Here's how the part is built. I have some questions about the finished solid (model axes, mm). Face numbers are marked on the shaded views. Coordinates: 2 decimals unless noted, no trailing zeros. Answer in a Markdown table with one row per item. Add a question column.
Item 1: Thinking about a two-plate mould opening in Z: for the marked faces 1 and 2, which applies, +Z half, -Z half, draft (parallel to the pull), parting line (faces both ways), or undercut?
Item 2: Will these pins go through, and if not, where does the flat tip stop? pin 1 Ø1.8 at (x, y) = (-30.08, -16.5) entering from -Z; pin 2 Ø3 at (x, y) = (28.5, 15) entering from -Z; pin 3 Ø3 at (x, y) = (-30.08, 16.5) entering from -Z.
Item 3: If I drill on line 1 along Y through (x, z) = (0, 0.2); line 2 along X through (y, z) = (-14, -0.3); line 3 along Y through (x, z) = (29.5, -0.4), over which ranges is the centre line in solid material (lowest first)? Write a range as from..to.
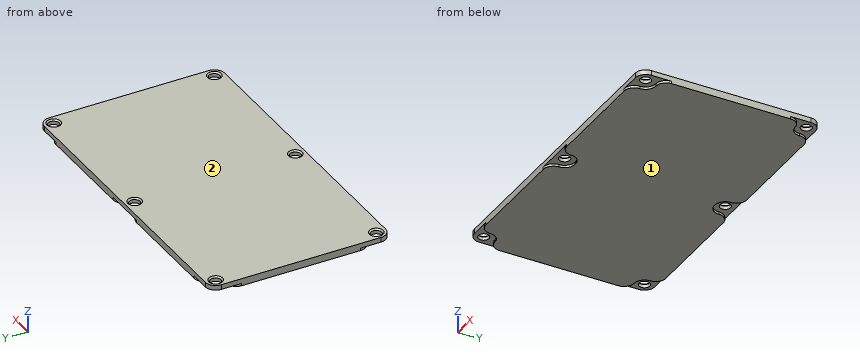
```python
from build123d import *

# Parameters (mm, degrees)
SKETCH_1_W          = 64
SKETCH_1_H          = 37
EXTRUDE_1_DEPTH     = 1
SKETCH_2_W          = 4.2
SKETCH_2_H          = 28.6
SKETCH_2_W_2        = 25.55
SKETCH_2_H_2        = 4.2
SKETCH_2_W_3        = 4.5
EXTRUDE_2_DEPTH     = 0.5
FILLET_1_R          = 2.1
CUT_EXTRUDE_1_REACH = 38.993
SKETCH_3_R          = 1.1
CHAMFER_1_SIZE      = 0.3


with BuildPart() as part:
    # 스케치1 → 보스-돌출1 (new body)
    with BuildSketch(Plane.XY):
        Rectangle(SKETCH_1_W, SKETCH_1_H)
    extrude(amount=EXTRUDE_1_DEPTH)

    # 스케치2 → 보스-돌출2 (add)
    with BuildSketch(Plane(origin=(0, 0, 0), x_dir=(-1, 0, 0), z_dir=(0, 0, -1))):
        with Locations((-29.9, 0)):
            Rectangle(SKETCH_2_W, SKETCH_2_H)
        with Locations((-15.025, 0)):
            Rectangle(SKETCH_2_W_2, SKETCH_2_H)
        with Locations((-15.025, 16.4)):
            Rectangle(SKETCH_2_W_2, SKETCH_2_H_2)
        with Locations((-15.025, -16.4)):
            Rectangle(SKETCH_2_W_2, SKETCH_2_H_2)
        with Locations((15.025, 0)):
            Rectangle(SKETCH_2_W_2, SKETCH_2_H)
        with Locations((15.025, 16.4)):
            Rectangle(SKETCH_2_W_2, SKETCH_2_H_2)
        Rectangle(SKETCH_2_W_3, SKETCH_2_H)
        with Locations((29.9, 0)):
            Rectangle(SKETCH_2_W, SKETCH_2_H)
        with Locations((15.025, -16.4)):
            Rectangle(SKETCH_2_W_2, SKETCH_2_H_2)
    extrude(amount=EXTRUDE_2_DEPTH)

    # 필렛1
    # the kernel refuses this fillet: 2.1 mm, written as the material it adds along each edge
    with BuildSketch(Plane(origin=(27.8, -14.3, 5.25), x_dir=(0, -1, 0), z_dir=(0, 0, -1))) as fillet_1_piece_1_section:
        with BuildLine():
            CenterArc((FILLET_1_R, -FILLET_1_R), FILLET_1_R, 90, 90)
            Line((0, -FILLET_1_R), (0, 0))
            Line((0, 0), (FILLET_1_R, 0))
        make_face()
    fillet_1_piece_1 = extrude(amount=5.75, mode=Mode.PRIVATE)
    fillet_1_piece_1 = split(fillet_1_piece_1, bisect_by=Plane(origin=(28.269072672, -14.769072672, 1), z_dir=(0, 0, -1)), keep=Keep.TOP, mode=Mode.PRIVATE)
    add(fillet_1_piece_1)
    with BuildSketch(Plane(origin=(-2.25, -14.3, 5.25), x_dir=(0, -1, 0), z_dir=(0, 0, -1))) as fillet_1_piece_2_section:
        with BuildLine():
            CenterArc((FILLET_1_R, -FILLET_1_R), FILLET_1_R, 90, 90)
            Line((0, -FILLET_1_R), (0, 0))
            Line((0, 0), (FILLET_1_R, 0))
        make_face()
    fillet_1_piece_2 = extrude(amount=5.75, mode=Mode.PRIVATE)
    fillet_1_piece_2 = split(fillet_1_piece_2, bisect_by=Plane(origin=(-1.780927328, -14.769072672, 1), z_dir=(0, 0, -1)), keep=Keep.TOP, mode=Mode.PRIVATE)
    add(fillet_1_piece_2)
    with BuildSketch(Plane(origin=(2.25, -14.3, 5.25), x_dir=(-1, 0, 0), z_dir=(0, 0, -1))) as fillet_1_piece_3_section:
        with BuildLine():
            CenterArc((FILLET_1_R, -FILLET_1_R), FILLET_1_R, 90, 90)
            Line((0, -FILLET_1_R), (0, 0))
            Line((0, 0), (FILLET_1_R, 0))
        make_face()
    fillet_1_piece_3 = extrude(amount=5.75, mode=Mode.PRIVATE)
    fillet_1_piece_3 = split(fillet_1_piece_3, bisect_by=Plane(origin=(1.780927328, -14.769072672, 1), z_dir=(0, 0, -1)), keep=Keep.TOP, mode=Mode.PRIVATE)
    add(fillet_1_piece_3)
    with BuildSketch(Plane(origin=(-27.8, -14.3, 5.25), x_dir=(-1, 0, 0), z_dir=(0, 0, -1))) as fillet_1_piece_4_section:
        with BuildLine():
            CenterArc((FILLET_1_R, -FILLET_1_R), FILLET_1_R, 90, 90)
            Line((0, -FILLET_1_R), (0, 0))
            Line((0, 0), (FILLET_1_R, 0))
        make_face()
    fillet_1_piece_4 = extrude(amount=5.75, mode=Mode.PRIVATE)
    fillet_1_piece_4 = split(fillet_1_piece_4, bisect_by=Plane(origin=(-28.269072672, -14.769072672, 1), z_dir=(0, 0, -1)), keep=Keep.TOP, mode=Mode.PRIVATE)
    add(fillet_1_piece_4)
    with BuildSketch(Plane(origin=(27.8, 14.3, 0), x_dir=(1, 0, 0), z_dir=(0, 0, -1)), Plane(origin=(-27.8, 14.3, 0), x_dir=(0, 1, 0), z_dir=(0, 0, -1))) as fillet_1_piece_5:
        with BuildLine():
            CenterArc((FILLET_1_R, -FILLET_1_R), FILLET_1_R, 90, 90)
            Line((0, -FILLET_1_R), (0, 0))
            Line((0, 0), (FILLET_1_R, 0))
        make_face()
    extrude(amount=0.5)
    with BuildSketch(Plane(origin=(-2.25, 14.3, 0), x_dir=(0, 1, 0), z_dir=(0, 0, -1)), Plane(origin=(2.25, 14.3, 0), x_dir=(-1, 0, 0), z_dir=(0, 0, -1))) as fillet_1_piece_6:
        with BuildLine():
            CenterArc((FILLET_1_R, FILLET_1_R), FILLET_1_R, 180, 90)
            Line((0, FILLET_1_R), (0, 0))
            Line((0, 0), (FILLET_1_R, 0))
        make_face()
    extrude(amount=0.5)
    # the kernel refuses this fillet: 2.1 mm, written as the material it takes off along each edge
    with BuildSketch(Plane(origin=(32, -18.5, -5.25), x_dir=(-1, 0, 0), z_dir=(0, 0, 1)), Plane(origin=(32, 18.5, -5.25), x_dir=(0, -1, 0), z_dir=(0, 0, 1))) as fillet_1_2_piece_1:
        with BuildLine():
            CenterArc((FILLET_1_R, -FILLET_1_R), FILLET_1_R, 90, 90)
            Line((0, -FILLET_1_R), (0, 0))
            Line((0, 0), (FILLET_1_R, 0))
        make_face()
    extrude(amount=11.5, mode=Mode.SUBTRACT)
    with BuildSketch(Plane(origin=(32, -14.3, 0), x_dir=(0, 1, 0), z_dir=(0, 0, -1)), Plane(origin=(27.8, 18.5, 0), x_dir=(-1, 0, 0), z_dir=(0, 0, -1)), Plane(origin=(-2.25, 18.5, 0), x_dir=(-1, 0, 0), z_dir=(0, 0, -1)), Plane(origin=(2.25, -18.5, 0), x_dir=(1, 0, 0), z_dir=(0, 0, -1)), Plane(origin=(-27.8, -18.5, 0), x_dir=(1, 0, 0), z_dir=(0, 0, -1)), Plane(origin=(-32, 14.3, 0), x_dir=(0, -1, 0), z_dir=(0, 0, -1))) as fillet_1_2_piece_2:
        with BuildLine():
            CenterArc((FILLET_1_R, -FILLET_1_R), FILLET_1_R, 90, 90)
            Line((0, -FILLET_1_R), (0, 0))
            Line((0, 0), (FILLET_1_R, 0))
        make_face()
    extrude(amount=5.75, mode=Mode.SUBTRACT)
    with BuildSketch(Plane(origin=(-32, -14.3, 0), x_dir=(0, 1, 0), z_dir=(0, 0, -1)), Plane(origin=(27.8, -18.5, 0), x_dir=(-1, 0, 0), z_dir=(0, 0, -1)), Plane(origin=(-2.25, -18.5, 0), x_dir=(-1, 0, 0), z_dir=(0, 0, -1)), Plane(origin=(2.25, 18.5, 0), x_dir=(1, 0, 0), z_dir=(0, 0, -1)), Plane(origin=(-27.8, 18.5, 0), x_dir=(1, 0, 0), z_dir=(0, 0, -1)), Plane(origin=(32, 14.3, 0), x_dir=(0, -1, 0), z_dir=(0, 0, -1))) as fillet_1_2_piece_3:
        with BuildLine():
            CenterArc((FILLET_1_R, FILLET_1_R), FILLET_1_R, 180, 90)
            Line((0, FILLET_1_R), (0, 0))
            Line((0, 0), (FILLET_1_R, 0))
        make_face()
    extrude(amount=5.75, mode=Mode.SUBTRACT)
    with BuildSketch(Plane(origin=(-32, -18.5, -5.25), x_dir=(1, 0, 0), z_dir=(0, 0, 1)), Plane(origin=(-32, 18.5, -5.25), x_dir=(0, -1, 0), z_dir=(0, 0, 1))) as fillet_1_2_piece_4:
        with BuildLine():
            CenterArc((FILLET_1_R, FILLET_1_R), FILLET_1_R, 180, 90)
            Line((0, FILLET_1_R), (0, 0))
            Line((0, 0), (FILLET_1_R, 0))
        make_face()
    extrude(amount=11.5, mode=Mode.SUBTRACT)

    # 스케치3 → 컷-돌출1 (cut, up to next)
    with BuildSketch(Plane.XY.offset(1), mode=Mode.PRIVATE) as cut_extrude_1_sk1:
        with Locations((-30.08, 16.5)):
            Circle(SKETCH_3_R)
    cut_extrude_1_tool1 = extrude(cut_extrude_1_sk1.sketch, amount=-CUT_EXTRUDE_1_REACH, mode=Mode.PRIVATE) & part.part
    # 스케치3 → 컷-돌출1 (cut, up to next)
    with BuildSketch(Plane.XY.offset(1), mode=Mode.PRIVATE) as cut_extrude_1_sk2:
        with Locations((0, 16.5)):
            Circle(SKETCH_3_R)
    cut_extrude_1_tool2 = extrude(cut_extrude_1_sk2.sketch, amount=-CUT_EXTRUDE_1_REACH, mode=Mode.PRIVATE) & part.part
    # 스케치3 → 컷-돌출1 (cut, up to next)
    with BuildSketch(Plane.XY.offset(1), mode=Mode.PRIVATE) as cut_extrude_1_sk3:
        with Locations((30.08, 16.5)):
            Circle(SKETCH_3_R)
    cut_extrude_1_tool3 = extrude(cut_extrude_1_sk3.sketch, amount=-CUT_EXTRUDE_1_REACH, mode=Mode.PRIVATE) & part.part
    # 스케치3 → 컷-돌출1 (cut, up to next)
    with BuildSketch(Plane.XY.offset(1), mode=Mode.PRIVATE) as cut_extrude_1_sk4:
        with Locations((30.08, -16.5)):
            Circle(SKETCH_3_R)
    cut_extrude_1_tool4 = extrude(cut_extrude_1_sk4.sketch, amount=-CUT_EXTRUDE_1_REACH, mode=Mode.PRIVATE) & part.part
    # 스케치3 → 컷-돌출1 (cut, up to next)
    with BuildSketch(Plane.XY.offset(1), mode=Mode.PRIVATE) as cut_extrude_1_sk5:
        with Locations((-30.08, -16.5)):
            Circle(SKETCH_3_R)
    cut_extrude_1_tool5 = extrude(cut_extrude_1_sk5.sketch, amount=-CUT_EXTRUDE_1_REACH, mode=Mode.PRIVATE) & part.part
    # 스케치3 → 컷-돌출1 (cut, up to next)
    with BuildSketch(Plane.XY.offset(1), mode=Mode.PRIVATE) as cut_extrude_1_sk6:
        with Locations((0, -16.5)):
            Circle(SKETCH_3_R)
    cut_extrude_1_tool6 = extrude(cut_extrude_1_sk6.sketch, amount=-CUT_EXTRUDE_1_REACH, mode=Mode.PRIVATE) & part.part
    add(cut_extrude_1_tool1.solids().sort_by_distance((-30.08, 16.5, 1))[0], mode=Mode.SUBTRACT)
    add(cut_extrude_1_tool2.solids().sort_by_distance((0, 16.5, 1))[0], mode=Mode.SUBTRACT)
    add(cut_extrude_1_tool3.solids().sort_by_distance((30.08, 16.5, 1))[0], mode=Mode.SUBTRACT)
    add(cut_extrude_1_tool4.solids().sort_by_distance((30.08, -16.5, 1))[0], mode=Mode.SUBTRACT)
    add(cut_extrude_1_tool5.solids().sort_by_distance((-30.08, -16.5, 1))[0], mode=Mode.SUBTRACT)
    add(cut_extrude_1_tool6.solids().sort_by_distance((0, -16.5, 1))[0], mode=Mode.SUBTRACT)

    # 모따기1
    chamfer_1_edges = [part.edges().sort_by_distance(p)[0] for p in [
        (-1.1, 16.5, 1),
        (28.98, 16.5, 1),
        (28.98, -16.5, 1),
        (-31.18, -16.5, 1),
        (-1.1, -16.5, 1),
        (-31.18, 16.5, 1),
    ]]
    chamfer(chamfer_1_edges, length=CHAMFER_1_SIZE)


solid = part.part
```
Values follow:
| question | item | result |
|---|---|---|
| 1 | face 1 | -Z half |
| 1 | face 2 | +Z half |
| 2 | pin 1 | passes through |
| 2 | pin 2 | stops at z = -0.5 |
| 2 | pin 3 | stops at z = 0 |
| 3 | line 1 | y = -18.5..-17.6, -15.4..15.4, 17.6..18.5 |
| 3 | line 2 | x = -30.98..30.98 |
| 3 | line 3 | y = -14.34..14.34 |
